Autodesk Inventor part; units mm, degrees
ref_plane "Plano de trabajo1" through (0, 0, 27) normal (0, 0, 1) x (1, 0, 0)
ref_plane "Plano de trabajo2" through (-44.5, -6, 27) normal (0, -1, 0) x (1, 0, 0)
ref_plane "Plano de trabajo3" through (-44.5, 6, 27) normal (0, 1, 0) x (1, 0, 0)
ref_plane "Plano de trabajo1" through (0, 0, 27) normal (0, 0, 1) x (1, 0, 0)
sketch "Boceto1" plane through (0, 0, 27) normal (0, 0, 1) x (1, 0, 0)
  arc A0 (0, -11) -> (-8.5797, 6.8839) centre (0, 0) ccw
  line L0 (0, -11) -> (-44.5, -11)
  line L1 (-46.5, -9) -> (-46.5, 1)
  line L2 (-44.5, 3) -> (-14.0947, 3)
  line L3 (-10.1948, 4.8709) -> (-8.5797, 6.8839)
  arc A1 (-14.0947, 3) -> (-10.1948, 4.8709) centre (-14.0947, 8) ccw
  arc A2 (-44.5, 3) -> (-46.5, 1) centre (-44.5, 1) ccw
  arc A3 (-46.5, -9) -> (-44.5, -11) centre (-44.5, -9) ccw
  circle A4 centre (0, 0) radius 2.5
  point P0 (-46.5, -11)
  point P1 (-46.5, 3)
  point P2 (11, 0)
  dimension "d1" = 22
  dimension "d3" = 5
  dimension "d4" = 14
  dimension "d5" = 57.5
  dimension "d6" = 2
  dimension "d7" = 5
extrude "Extrusión1" add sketch "Boceto1" along normal blind 3
mirror "Simetría1" about plane through (0, 0, 0) normal (0, 0, 1) of "Extrusión1"
ref_plane "Plano de trabajo2" through (-44.5, -6, 27) normal (0, -1, 0) x (1, 0, 0)
sketch "Boceto2" plane through (-44.5, -6, 27) normal (0, -1, 0) x (1, 0, 0)
  line L0 (0, 0) -> (44.5, 0)
  line L1 (23, 0) -> (-10.5, 0)
  line L2 (-12.5, -2) -> (-12.5, -52)
  line L3 (-10.5, -54) -> (23, -54)
  line L4 (0, -54) -> (44.5, -54)
  line L5 (21.6267, -49.5581) -> (14, -41.5219)
  line L6 (14, -41.5219) -> (14, -12.4781)
  line L7 (14, -12.4781) -> (21.6267, -4.4419)
  line L8 (23, -1) -> (23, 0)
  line L9 (23, -53) -> (23, -54)
  line L10 (0, 3) -> (-2, 3)
  line L11 (14, -27) -> (-19.9317, -27) construction
  arc A0 (21.6267, -4.4419) -> (23, -1) centre (18, -1) ccw
  arc A1 (23, -53) -> (21.6267, -49.5581) centre (18, -53) ccw
  arc A2 (-10.5, 0) -> (-12.5, -2) centre (-10.5, -2) ccw
  arc A3 (-12.5, -52) -> (-10.5, -54) centre (-10.5, -52) ccw
  point P0 (44.5, -27)
  point P1 (-12.5, 0)
  point P2 (-12.5, -54)
  point P3 (-1, 3)
  dimension "d11" = 26.5
  dimension "d12" = 11.5
  dimension "d13" = 9
  dimension "d14" = 9
  dimension "d16" = 5
  dimension "d17" = 1
  dimension "d18" = 1
  dimension "d19" = 27
  dimension "d40" = 2
extrude "Extrusión2" add sketch "Boceto2" along normal blind 3
ref_plane "Plano de trabajo3" through (-44.5, 6, 27) normal (0, 1, 0) x (1, 0, 0)
sketch "Boceto3" plane through (-44.5, 6, 27) normal (0, 1, 0) x (1, 0, 0)
  line L0 (-10.5, 44.5) -> (17.5, 44.5)
  line L1 (19.5, 42.5) -> (19.5, 11.5)
  line L2 (17.5, 9.5) -> (-10.5, 9.5)
  line L3 (-12.5, 11.5) -> (-12.5, 42.5)
  line L4 (0, 27) -> (-59, 27) construction
  line L5 (30.4053, 0) -> (0, 0)
  arc A0 (-10.5, 44.5) -> (-12.5, 42.5) centre (-10.5, 42.5) ccw
  arc A1 (-12.5, 11.5) -> (-10.5, 9.5) centre (-10.5, 11.5) ccw
  arc A2 (17.5, 9.5) -> (19.5, 11.5) centre (17.5, 11.5) ccw
  arc A3 (19.5, 42.5) -> (17.5, 44.5) centre (17.5, 42.5) ccw
  line L6 (-12.5, 2) -> (-12.5, 52) construction
  point P0 (44.5, 27)
  point P1 (-12.5, 44.5)
  point P2 (19.5, 44.5)
  point P3 (-12.5, 9.5)
  point P4 (-12.5, 27)
  point P5 (-12.5, 0)
  point P6 (-12.5, 54)
  dimension "d23" = 35
  dimension "d24" = 32
  dimension "d25" = 27
  dimension "d26" = 2
extrude "Extrusión3" add sketch "Boceto3" along normal blind 3
sketch "Boceto4" plane through (-44.5, 9, 27) normal (0, 1, 0) x (1, 0, 0)
  line L0 (-12.5, 42.5) -> (-12.5, 11.5) construction
  line L1 (-12.5, 27) -> (20, 27) construction
  circle A0 centre (8.5, 38.75) radius 2.5
  circle A1 centre (-1.5, 38.75) radius 2.5
  line L2 (3.5, 27) -> (3.5, -23) construction
  circle A2 centre (8.5, 15.25) radius 2.5
  circle A3 centre (-1.5, 15.25) radius 2.5
  point P0 (44.5, 27)
  dimension "d29" = 5
  dimension "d30" = 10
  dimension "d31" = 16
  dimension "d32" = 11.75
extrude "Extrusión4" cut sketch "Boceto4" against normal up to surface (18 mm away)
fillet "Empalme1" radius 15 2 edges at (-30.5, -7.5, 14.5219) (-30.5, -7.5, -14.5219)
sketch "Boceto5" plane through (0, 0, 30) normal (0, 0, 1) x (1, 0, 0)
  line L0 (-34, -8) -> (-34, 17.5513) construction
  line L1 (-34, 17.5513) -> (-23.3891, 17.5513) construction
  line L2 (-23.3891, 17.5513) -> (-23.3891, -8) construction
  line L3 (-23.3891, -8) -> (-34, -8) construction
  spline S0 degree 2 poles (-25.812, 0.1491) (-24.9465, 0.1491) (-23.4684, -0.4052) (-22.9238, -0.9109) knots 0 0 0 1 2 2 2
  spline S1 degree 2 poles (-22.9238, -0.9109) (-22.3793, -1.4165) (-21.7472, -2.9238) (-21.7472, -3.8574) knots 0 0 0 1 2 2 2
  spline S2 degree 2 poles (-21.7472, -3.8574) (-21.7472, -4.7131) (-22.1264, -6.3857) (-22.4279, -6.9984) knots 0 0 0 1 2 2 2
  line L4 (-22.4279, -6.9984) -> (-24.1297, -6.9984)
  line L5 (-24.1297, -6.9984) -> (-24.1297, -6.8817)
  spline S3 degree 2 poles (-24.1297, -6.8817) (-23.9935, -6.6969) (-23.6434, -6.0065) (-23.4878, -5.5883) knots 0 0 0 1 2 2 2
  spline S4 degree 2 poles (-23.4878, -5.5883) (-23.3225, -5.1118) (-23.1378, -4.3241) (-23.1378, -3.8282) knots 0 0 0 1 2 2 2
  spline S5 degree 2 poles (-23.1378, -3.8282) (-23.1378, -3.342) (-23.4878, -2.4279) (-23.8671, -2.0972) knots 0 0 0 1 2 2 2
  spline S6 degree 2 poles (-23.8671, -2.0972) (-24.2269, -1.7958) (-25.1799, -1.4846) (-25.8217, -1.4846) knots 0 0 0 1 2 2 2
  spline S7 degree 2 poles (-25.8217, -1.4846) (-26.4635, -1.4846) (-27.2804, -1.8347) (-27.5527, -2.1653) knots 0 0 0 1 2 2 2
  spline S8 degree 2 poles (-27.5527, -2.1653) (-27.8541, -2.5057) (-28.107, -3.517) (-28.107, -4.1297) knots 0 0 0 1 2 2 2
  spline S9 degree 2 poles (-28.107, -4.1297) (-28.107, -4.7909) (-27.9028, -6.1037) (-27.8152, -6.5024) knots 0 0 0 1 2 2 2
  line L6 (-27.8152, -6.5024) -> (-34, -6.5024)
  line L7 (-34, -6.5024) -> (-34, 0.081)
  line L8 (-34, 0.081) -> (-32.59, 0.081)
  line L9 (-32.59, 0.081) -> (-32.59, -4.9562)
  line L10 (-32.59, -4.9562) -> (-29.3906, -4.9562)
  spline S10 degree 2 poles (-29.3906, -4.9562) (-29.4295, -4.6645) (-29.4587, -4.1005) (-29.4587, -3.8671) knots 0 0 0 1 2 2 2
  spline S11 degree 2 poles (-29.4587, -3.8671) (-29.4587, -2.9433) (-29.1572, -1.6694) (-28.7099, -1.0859) knots 0 0 0 1 2 2 2
  spline S12 degree 2 poles (-28.7099, -1.0859) (-28.2626, -0.4927) (-26.9011, 0.1491) (-25.812, 0.1491) knots 0 0 0 1 2 2 2
  point P0 (0, 0)
extrude "Extrusión5" cut sketch "Boceto5" against normal blind 0.5
ref_plane "Plano de trabajo4" through (-44.5, 0, 27) normal (0, -1, 0) x (1, 0, 0)
sketch "Boceto6" plane through (-44.5, 0, 27) normal (0, -1, 0) x (1, 0, 0)
  circle A0 centre (8.5, -15.25) radius 2.5
  circle A1 centre (-1.5, -15.25) radius 2.5
  circle A2 centre (8.5, -38.75) radius 2.5
  circle A3 centre (-1.5, -38.75) radius 2.5
  point P0 (44.5, -27)
extrude "Extrusión6" add sketch "Boceto6" along normal mid plane 18
equation "\"Radio_pliegue\" = Grosor"
equation "\"Anchura_desahogo_plegado\" = Grosor"
equation "\"Profundidad_desahogo_plegado\" = 0.5 * Grosor"
equation "\"Tamaño_destalonado\" = 4 * Grosor"
equation "\"Remanente_mínimo\" = 2 * Grosor"
equation "\"Radiodetransición\" = Radio_pliegue"
equation "\"Tamaño_de_radio_de_Jacobi\" = Radio_pliegue"
equation "\"TamañoSeparación\" = Grosor"
Geometry check sheet. Reference: the model listing, model coordinates, mm. A direction names the side the tool comes from. Round coordinates to 2 decimals unless told otherwise and drop trailing zeros. Loops run counter-clockwise (first coordinate to the right, second up) from the corner with the lowest first, then second, coordinate; pieces in that order, holes last.
Item 1: Cross-section at B-B on x = -36. Record the boundary of the cut face in (y, z).
Item 2: Mould release check, pull along Y, two halves, no side actions. Record for faces 1 (the cylindrical face through (-43.69, 0.08, 12.71)), 2 (the flat face through (-23, -11, -28)), 3 (the cylindrical face through (-33.69, 0.08, 12.71)), 4 (the cylindrical face through (-56.43, -7.48, 26.4)): pulls with the +Y half, pulls with the -Y half, needs draft (parallel to the pull), parting line crosses it, or undercut.
Item 3: Cross-section at C-C on x = -13. Record the boundary of the cut face in (y, z).
Item 4: Cross-section at A-A on z = 3.5. Record the boundary of the cut face in (x, y), then the cut area to 4 significant figures.
Item 5: Thickness scan on line 1 (Y direction, x = 0, z = -28.3); line 2 (Z direction, x = -19, y = -3.75); line 3 (Y direction, x = -48, z = 1). Record the ranges inside material, lowest first.
Item 6: Gauge pin test, flat ends, axial feed: pin 1 (3.5 mm diameter, centred on y = 7, z = -1, fed in from +X); pin 2 (1.5 mm diameter, centred on x = -29, z = -28.5, fed in from +Y); pin 3 (10.5 mm diameter, centred on x = -33, z = 6, fed in from +Y); pin 4 (10 mm diameter, centred on x = -16, z = 15, fed in from +Y). Record the tip position at first contact, or that the pin passes through.
Item 7: Cross-section at D-D on y = 1.75. Record the boundary of the cut face in (x, z).
Item 8: Access from +Z, -Z, +X, -X, +Y, -Y to the whole of each face (thin tool, end or side, straight path). Record for faces 5 (the cylindrical face through (-33.69, 0.08, -10.79)), 6 (the cylindrical face through (-56.43, 7.48, -16.9)), 7 (the flat face through (-30.5, -7, 0)), 8 (the flat face through (-51, -7, 27)).
Answer sheet:
1. outline: (-11, -30) - (3, -30) - (3, -27) - (-6, -27) - (-6, -14.25) - (6, -14.25) - (6, -17.5) - (9, -17.5) - (9, 17.5) - (6, 17.5) - (6, 14.25) - (-6, 14.25) - (-6, 27) - (3, 27) - (3, 30) - (-11, 30) - (-11, 27) - (-9, 27) - (-9, -27) - (-11, -27) - close; hole (-6, -9.25) - (6, -9.25) - (6, 9.25) - (-6, 9.25) - close
2. face 1: undercut
2. face 2: pulls with the -Y half
2. face 3: undercut
2. face 4: needs draft
3. outline: (-11, -30) - (3.12, -30) - (3.12, -27) - (-11, -27) - close; (-11, 27) - (3.12, 27) - (3.12, 30) - (-11, 30) - close
4. outline: (-57, -9) - (-30.5, -9) - (-30.5, -6) - (-57, -6) - close; (-57, 6) - (-25, 6) - (-25, 9) - (-57, 9) - close
4. area: 175.5 mm2
5. line 1: y = -11 to -2.5, 2.5 to 11
5. line 2: z = -30 to -27, 27 to 30
5. line 3: y = -9 to -6, 6 to 9
6. pin 1: stops at x = -25
6. pin 2: stops at y = 3
6. pin 3: stops at y = 9
6. pin 4: passes through
7. outline: circle Ø5 at (-46, -11.75); circle Ø5 at (-46, 11.75); (-46.35, -30) - (-1.79, -30) - (-1.79, -27) - (-46.35, -27) - close; (-46.35, 27) - (-1.79, 27) - (-1.79, 30) - (-46.35, 30) - close; circle Ø5 at (-36, -11.75); circle Ø5 at (-36, 11.75); (1.79, -30) - (10.86, -30) - (10.86, -27) - (1.79, -27) - close; (1.79, 27) - (10.86, 27) - (10.86, 30) - (1.79, 30) - close
8. face 5: none
8. face 6: -Z, -X, +Y
8. face 7: +X, -Y
8. face 8: +Z, -X, +Y, -Y
